```python
from build123d import *

# Parameters (mm, degrees)
SKETCH1_W           = 50.8
SKETCH1_H           = 50.8
BOSS_EXTRUDE1_DEPTH = 6.35
FILLET1_R           = 6.35
BOSS_EXTRUDE2_START = 19.05
BOSS_EXTRUDE2_DEPTH = 19.05
SKETCH5_W           = 50.8
SKETCH5_H           = 50.8
BOSS_EXTRUDE3_DEPTH = 6.35
FILLET2_R           = 6.35
SKETCH6_R           = 3.175
BOSS_EXTRUDE4_DEPTH = 12.7
BOSS_EXTRUDE5_DEPTH = 19.05
SKETCH8_R           = 0.635
CUT_EXTRUDE2_DEPTH  = 2.54


with BuildPart() as part:
    # Sketch1 → Boss-Extrude1 (new body)
    with BuildSketch(Plane(origin=(0, 0, 0), x_dir=(1, 0, 0), z_dir=(0, 1, 0))):
        with Locations((25.4, 25.4)):
            Rectangle(SKETCH1_W, SKETCH1_H)
    extrude(amount=BOSS_EXTRUDE1_DEPTH)

    # Fillet1
    fillet1_edges = [part.edges().sort_by_distance(p)[0] for p in [
        (0, 3.175, -50.8),
        (50.8, 3.175, -50.8),
        (50.8, 3.175, 0),
        (0, 3.175, 0),
    ]]
    fillet(fillet1_edges, radius=FILLET1_R)

    # Sketch3 → Boss-Extrude2 (add)
    with BuildSketch(Plane(origin=(0, 6.35, 0), x_dir=(1, 0, 0), z_dir=(0, 1, 0)).offset(BOSS_EXTRUDE2_START)):
        with BuildLine():
            Line((11.43, 48.26), (39.37, 48.26))
            ThreePointArc((39.37, 48.26), (48.940128061, 48.940128061), (48.26, 39.37))
            Line((48.26, 39.37), (48.26, 11.43))
            ThreePointArc((48.26, 11.43), (48.940128061, 1.859871939), (39.37, 2.54))
            Line((39.37, 2.54), (11.43, 2.54))
            ThreePointArc((11.43, 2.54), (1.859871939, 1.859871939), (2.54, 11.43))
            Line((2.54, 11.43), (2.54, 39.37))
            ThreePointArc((2.54, 39.37), (1.859871939, 48.940128061), (11.43, 48.26))
        make_face()
    extrude(amount=-BOSS_EXTRUDE2_DEPTH)

    # Sketch5 → Boss-Extrude3 (add)
    with BuildSketch(Plane(origin=(0, 25.4, 0), x_dir=(1, 0, 0), z_dir=(0, 1, 0))):
        with Locations((25.4, 25.4)):
            Rectangle(SKETCH5_W, SKETCH5_H)
    extrude(amount=BOSS_EXTRUDE3_DEPTH)

    # Fillet2
    fillet2_edges = [part.edges().sort_by_distance(p)[0] for p in [
        (50.8, 28.575, -50.8),
        (0, 28.575, -50.8),
        (50.8, 28.575, 0),
        (0, 28.575, 0),
    ]]
    fillet(fillet2_edges, radius=FILLET2_R - 0.0001)  # a hair under: the kernel refuses the full size

    # Sketch6 → Boss-Extrude4 (add)
    with BuildSketch(Plane(origin=(0, 31.75, 0), x_dir=(1, 0, 0), z_dir=(0, 1, 0))):
        with Locations(Location((25.4, 25.4, 0), (0, 0, 270))):
            Circle(SKETCH6_R)
    extrude(amount=BOSS_EXTRUDE4_DEPTH)

    # Sketch7 → Boss-Extrude5 (add)
    with BuildSketch(Plane(origin=(0, 44.45, 0), x_dir=(1, 0, 0), z_dir=(0, 1, 0))):
        with BuildLine():
            Line((28.575, 26.035), (28.575, 24.765))
            Line((28.575, 24.765), (26.854967783, 24.765))
            ThreePointArc((26.854967783, 24.765), (23.8125, 25.4), (26.854967783, 26.035))
            Line((26.854967783, 26.035), (28.575, 26.035))
        make_face()
    extrude(amount=BOSS_EXTRUDE5_DEPTH)

    # Sketch8 → Cut-Extrude2 (cut)
    with BuildSketch(Plane.XY.offset(-24.765)):
        with Locations((27.715591, 52.07)):
            Circle(SKETCH8_R)
        with Locations((27.715591, 57.15)):
            Circle(SKETCH8_R)
    extrude(amount=-CUT_EXTRUDE2_DEPTH, mode=Mode.SUBTRACT)


solid = part.part
```
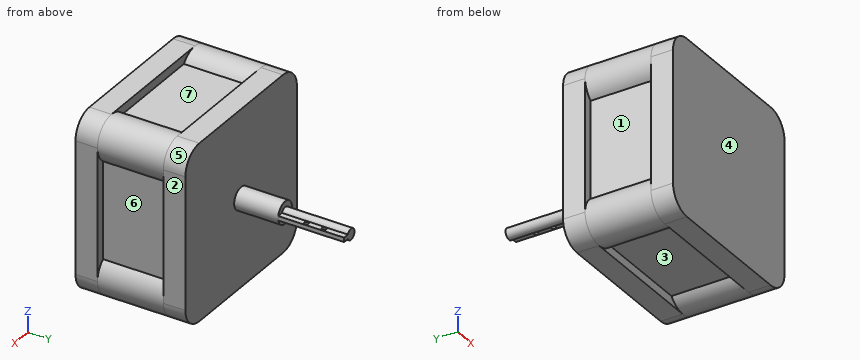
CAD build for the part. Positions are in the model's coordinates, mm. Face numbers are marked on the shaded views. A direction names the side the tool comes from. Round coordinates to 2 decimals unless told otherwise and drop trailing zeros. Loops run counter-clockwise (first coordinate to the right, second up) from the corner with the lowest first, then second, coordinate; pieces in that order, holes last. Notation, with made-up numbers: M 8.5,53.25 L 37.5,53.25 A22 cw 37.5,74.25 Z; hole C -33.5,40 d2. An arc over 180 degrees is marked long. Return JSON: item names as keys, results as strings. Group by question number.
(1) Saw through at A-A, the plane z = -18. List the corners of the cut face in (x, y), and give its area (3 significant figures).
(2) Wall check: probe 1 along X at (y, z) = (57.15, -25.5) (3 decimals); probe 2 along Y at (x, z) = (34.5, -41.5); probe 3 along Y at (x, z) = (21, -48.5). Give the ranges that are in metal, low to high. Write a range as [from, to].
(3) Saw through at D-D, the plane x = 42. List the corners of the cut face in (y, z), and give its area (3 significant figures).
(4) Saw through at B-B, the plane y = 9.5. List the corners of the cut face in (x, z).
(5) Tool access for the marked faces 1, 2 and 3: list every direction of +Z, -Z, +X, -X, +Y, -Y with a clear straight run to the whole face (end or side of a thin tool).
(6) Drop flat-ended pins along their axis: P1, Ø5, axis at x = 11, z = -36.5, coming from the +Y side; P2, Ø3, axis at x = 27, y = 9.5, coming from the -Z side; P3, Ø4, axis at x = 12, y = 11, coming from the +Z side. Give the stop position or say it passes through.
(7) Mould opens along Y. For the marked faces 4, 5, 6 and 7 say: +Y half, -Y half, draft (parallel to the pull), parting line (faces both ways), or undercut.
Answer list:
{
 "1": {"outline": "M 0,0 L 50.8,0 L 50.8,6.35 L 48.26,6.35 L 48.26,25.4 L 50.8,25.4 L 50.8,31.75 L 0,31.75 L 0,25.4 L 2.54,25.4 L 2.54,6.35 L 0,6.35 Z", "area": "1,520 mm2"},
 "2": {"probe 1": "[23.816, 27.081], [28.351, 28.575]", "probe 2": "[0, 31.75]", "probe 3": "[0, 6.35], [25.4, 31.75]"},
 "3": {"outline": "M 0,-50.8 L 6.35,-50.8 L 6.35,-50.31 L 25.4,-50.31 L 25.4,-50.8 L 31.75,-50.8 L 31.75,0 L 25.4,0 L 25.4,-0.49 L 6.35,-0.49 L 6.35,0 L 0,0 Z", "area": "1,590 mm2"},
 "4": {"outline": "M 2.54,-39.37 A6.35 ccw long 11.43,-48.26 L 39.37,-48.26 A6.35 ccw long 48.26,-39.37 L 48.26,-11.43 A6.35 ccw long 39.37,-2.54 L 11.43,-2.54 A6.35 ccw long 2.54,-11.43 Z"},
 "5": {"face 1": "-X", "face 2": "+Z, -Z, +X, +Y, -Y", "face 3": "-Z"},
 "6": {"P1": "y = 31.75", "P2": "z = -48.26", "P3": "z = -1.15"},
 "7": {"face 4": "-Y half", "face 5": "draft", "face 6": "undercut", "face 7": "undercut"}
}
